Part model, mm, in its own coordinate system. A direction names the side the tool comes from. Round coordinates to 2 decimals unless told otherwise and drop trailing zeros. Loops run counter-clockwise (first coordinate to the right, second up) from the corner with the lowest first, then second, coordinate; pieces in that order, holes last.
(1) Probe probe 1 along X at (y, z) = (12.8, 0); probe 2 along X at (y, z) = (2.55, 0) (3 decimals); probe 3 along Y at (x, z) = (14, 17.5). List the from-to ranges inside material, lowest first.
(2) Cut at B-B on x = 0. List the corners of the cut face in (y, z).
(3) Cut at D-D on z = -22. List the corners of the cut face in (x, y).
(4) Cut at C-C on y = 15. List the corners of the cut face in (x, z), then the cut area to 3 significant figures.
(5) Cut at A-A on z = 0. List the corners of the cut face in (x, y) (3 decimals).
(6) Mould opens along Z. For faces 4 (the face through (-30, 2, 10)), 5 (the face through (12, 5, 15)), 6 (the face through (6, 11, 10)) say: +Z half, -Z half, draft (parallel to the pull), parting line (faces both ways), or undercut.
(7) Flat gauge pins, fed straight in: pin 1 (1 mm diameter, centred on x = 3, y = 2.5, fed in from -Z); pin 2 (20 mm diameter, centred on x = 0, z = -2, fed in from -Y); pin 3 (2.5 mm diameter, centred on x = -28.5, y = 3.5, fed in from -Z); pin 4 (22.5 mm diameter, centred on x = 0, z = 0, fed in from -Y). Where does each tip first touch, or does it go through?
(8) Tool access for faces 1 (the face through (29, 2, 10)), 2 (the face through (-13.18, 13.46, -2.93)), 3 (the face through (-11, 5, 4)): list every direction of +Z, -Z, +X, -X, +Y, -Y with a clear straight run to the whole face (end or side of a thin tool).
from build123d import *

# Parameters (mm, degrees)
SKETCH1_R           = 12.5
BOSS_EXTRUDE1_DEPTH = 5
SKETCH2_R           = 16.5
SKETCH2_R_2         = 11.5
BOSS_EXTRUDE2_DEPTH = 6
SKETCH3_R           = 16.5
SKETCH3_R_2         = 13.5
BOSS_EXTRUDE3_DEPTH = 5
FILLET1_R           = 2.5
FILLET2_R           = 5


with BuildPart() as part:
    # Sketch1 → Boss-Extrude1 (new body)
    with BuildSketch(Plane(origin=(0, 0, 0), x_dir=(1, 0, 0), z_dir=(0, 1, 0))):
        with BuildLine():
            Line((-22.912878475, 10), (-32.945, 10))
            Line((-32.945, 10), (-32.945, -10))
            Line((-32.945, -10), (-22.912878475, -10))
            ThreePointArc((-22.912878475, -10), (0, -25), (22.912878475, -10))
            Line((22.912878475, -10), (32.945, -10))
            Line((32.945, -10), (32.945, 10))
            Line((32.945, 10), (22.912878475, 10))
            ThreePointArc((22.912878475, 10), (0, 25), (-22.912878475, 10))
        make_face()
        with Locations(Location((0, 0, 0), (0, 0, 270))):
            Circle(SKETCH1_R, mode=Mode.SUBTRACT)
    extrude(amount=BOSS_EXTRUDE1_DEPTH)

    # Sketch2 → Boss-Extrude2 (add)
    with BuildSketch(Plane(origin=(0, 5, 0), x_dir=(1, 0, 0), z_dir=(0, 1, 0))):
        with Locations(Location((0, 0, 0), (0, 0, 270))):
            Circle(SKETCH2_R)
        with Locations(Location((0, 0, 0), (0, 0, 270))):
            Circle(SKETCH2_R_2, mode=Mode.SUBTRACT)
    extrude(amount=BOSS_EXTRUDE2_DEPTH)

    # Sketch3 → Boss-Extrude3 (add)
    with BuildSketch(Plane(origin=(0, 11, 0), x_dir=(1, 0, 0), z_dir=(0, 1, 0))):
        with Locations(Location((0, 0, 0), (0, 0, 270))):
            Circle(SKETCH3_R)
        with Locations(Location((0, 0, 0), (0, 0, 270))):
            Circle(SKETCH3_R_2, mode=Mode.SUBTRACT)
    extrude(amount=BOSS_EXTRUDE3_DEPTH)

    # Fillet1
    fillet1_edges = [part.edges().sort_by_distance(p)[0] for p in [
        (0, 5, -16.5),
    ]]
    fillet(fillet1_edges, radius=FILLET1_R)

    # Fillet2
    fillet2_edges = [part.edges().sort_by_distance(p)[0] for p in [
        (-22.912878475, 2.5, -10),
        (22.912878475, 2.5, -10),
        (22.912878475, 2.5, 10),
        (-22.912878475, 2.5, 10),
    ]]
    fillet(fillet2_edges, radius=FILLET2_R)


solid = part.part
Final values:
1. probe 1: x = -16.5 to -13.5, 13.5 to 16.5
1. probe 2: x = -32.945 to -12.5, 12.5 to 32.945
1. probe 3: y = 0 to 5
2. outline: (0, -25) - (5, -25) - (5, -19) arc R2.5 cw to (7.5, -16.5) - (16, -16.5) - (16, -13.5) - (11, -13.5) - (11, -11.5) - (5, -11.5) - (5, -12.5) - (0, -12.5) - close; (0, 12.5) - (5, 12.5) - (5, 11.5) - (11, 11.5) - (11, 13.5) - (16, 13.5) - (16, 16.5) - (7.5, 16.5) arc R2.5 cw to (5, 19) - (5, 25) - (0, 25) - close
3. outline: (-11.87, 0) - (11.87, 0) - (11.87, 5) - (-11.87, 5) - close
4. outline: circle Ø33 at (0, 0); hole circle Ø27 at (0, 0)
4. area: 283 mm2
5. outline: (-32.945, 0) - (-12.5, 0) - (-12.5, 5) - (-11.5, 5) - (-11.5, 11) - (-13.5, 11) - (-13.5, 16) - (-16.5, 16) - (-16.5, 7.5) arc R2.5 cw to (-19, 5) - (-32.945, 5) - close; (11.5, 5) - (12.5, 5) - (12.5, 0) - (32.945, 0) - (32.945, 5) - (19, 5) arc R2.5 cw to (16.5, 7.5) - (16.5, 16) - (13.5, 16) - (13.5, 11) - (11.5, 11) - close
6. face 4: +Z half
6. face 5: draft
6. face 6: undercut
7. pin 1: stops at z = -24.87
7. pin 2: stops at y = 5
7. pin 3: stops at z = -10
7. pin 4: passes through
8. face 1: +Z, +X, +Y, -Y
8. face 2: +Y
8. face 3: -Y
